Could you check a few things on this model? Use its own coordinates, in mm. Face numbers are marked on the shaded views. A direction names the side the tool comes from. Round coordinates to 2 decimals unless told otherwise and drop trailing zeros. Loops run counter-clockwise (first coordinate to the right, second up) from the corner with the lowest first, then second, coordinate; pieces in that order, holes last. Notation, with made-up numbers: (-4.5, 58) -> (45.5, 58) arc R22 ccw to (45.5, 79) -> close; hole circle Ø7 at (79, -25). An arc over 180 degrees is marked (long way). One line per item, written item: value.
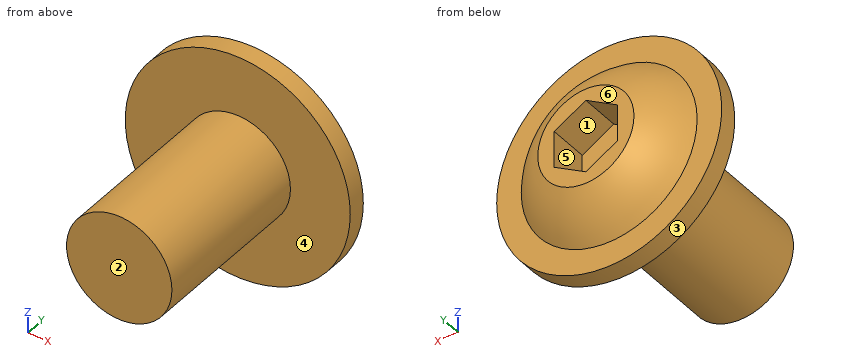
```python
from build123d import *

# Parameters (mm, degrees)
SKETCH1_R           = 3.96875
BOSS_EXTRUDE1_DEPTH = 12.7
SKETCH2_R           = 8.475
BOSS_EXTRUDE2_DEPTH = 1.4
CUT_EXTRUDE1_DEPTH  = 3


with BuildPart() as part:
    # Sketch1 → Boss-Extrude1 (new body)
    with BuildSketch(Plane(origin=(0, 0, 0), x_dir=(1, 0, 0), z_dir=(0, 1, 0))):
        Circle(SKETCH1_R)
    extrude(amount=BOSS_EXTRUDE1_DEPTH)

    # Sketch2 → Boss-Extrude2 (add)
    with BuildSketch(Plane(origin=(0, 12.7, 0), x_dir=(1, 0, 0), z_dir=(0, 1, 0))):
        Circle(SKETCH2_R)
    extrude(amount=BOSS_EXTRUDE2_DEPTH)

    # Sketch3 → Revolve2 (revolve)
    with BuildSketch(Plane.XY):
        with BuildLine():
            Line((-3.625, 16.6), (0, 16.6))
            Line((0, 16.6), (0, 14.1))
            Line((0, 14.1), (-6.625, 14.1))
            ThreePointArc((-6.625, 14.1), (-5.275236962, 15.530284354), (-3.625, 16.6))
        make_face()
    revolve(axis=Axis((0, 16.6, 0), (0, -1, 0)))

    # Sketch4 → Cut-Extrude1 (cut)
    with BuildSketch(Plane(origin=(0, 16.6, 0), x_dir=(1, 0, 0), z_dir=(0, 1, 0))):
        Polygon((-2.38125, 1.374815329), (-2.38125, -1.374815329), (0, -2.749630657), (2.38125, -1.374815329), (2.38125, 1.374815329), (0, 2.749630657), align=None)
    extrude(amount=-CUT_EXTRUDE1_DEPTH, mode=Mode.SUBTRACT)


solid = part.part
```
Item 1: I need wall thicknesses on line 1 (Y direction, x = -1, z = 1); line 2 (Y direction, x = 2, z = 7.5); line 3 (Z direction, x = 0.75, y = 3.25). Which ranges of each line are inside material? Lowest first, please. Write a range as from..to.
Output:
line 1: y = 0..13.6
line 2: y = 12.7..14.1
line 3: z = -3.9..3.9
Item 2: If we mould it in two halves opening along X, with no side actions, what happens to the marked faces 1, 2 and 3? For each: released by +X, released by -X, zero draft, split by the parting line, or undercut.
Output:
face 1: undercut
face 2: zero draft
face 3: split by the parting line
Item 3: If we section it at C-C on y = 14.5: List the corners of the cut face in (x, z) for me.
Output:
outline: circle Ø12.62 at (0, 0); hole (-2.38, -1.37) -> (0, -2.75) -> (2.38, -1.37) -> (2.38, 1.37) -> (0, 2.75) -> (-2.38, 1.37) -> close
Item 4: Will these pins go through, and if not, where does the flat tip stop? pin 1 Ø1.4 at (y, z) = (15.5, 0) entering from -X; pin 2 Ø5 at (y, z) = (15, -4) entering from +X; pin 3 Ø1 at (x, z) = (-3.5, 5.5) entering from -Y.
Output:
pin 1: stops at x = -6.04
pin 2: stops at x = 8.31
pin 3: stops at y = 12.7
Item 5: If we section it at D-D on y = 2: List the corners of the cut face in (x, z) for me, plus the area to 3 significant figures.
Output:
outline: circle Ø7.94 at (0, 0)
area: 49.5 mm²
Item 6: If we section it at B-B on z = 2: List the corners of the cut face in (x, y) for me.
Output:
outline: (-8.24, 12.7) -> (-3.43, 12.7) -> (-3.43, 0) -> (3.43, 0) -> (3.43, 12.7) -> (8.24, 12.7) -> (8.24, 14.1) -> (6.32, 14.1) arc R7.99 ccw to (3.02, 16.6) -> (1.3, 16.6) -> (1.3, 13.6) -> (-1.3, 13.6) -> (-1.3, 16.6) -> (-3.02, 16.6) arc R7.99 ccw to (-6.32, 14.1) -> (-8.24, 14.1) -> close
Item 7: For the marked faces 4, 5 and 6, which set-ups out of +Z, -Z, +X, -X, +Y, -Y let a thin tool reach every point of the face, with its end or its side?
Output:
face 4: -Y
face 5: +Y
face 6: +Z, -Z, +X, -X, +Y
Item 8: If we section it at A-A on x = 1.25: List the corners of the cut face in (y, z) for me, plus the area to 3 significant figures.
Output:
outline: (0, -3.77) -> (12.7, -3.77) -> (12.7, -8.38) -> (14.1, -8.38) -> (14.1, -6.51) arc R8.14 ccw to (16.6, -3.4) -> (16.6, -2.03) -> (13.6, -2.03) -> (13.6, 2.03) -> (16.6, 2.03) -> (16.6, 3.4) arc R8.14 ccw to (14.1, 6.51) -> (14.1, 8.38) -> (12.7, 8.38) -> (12.7, 3.77) -> (0, 3.77) -> close
area: 133 mm²
